Verification items for this drawing (mm, ordinates from the low corner). Coordinates: 2 decimals unless noted, no trailing zeros. Order: outer loops, then holes, each group sorted by start corner. A loop starts at its lowest first (then second) coordinate and runs counter-clockwise, first axis right, second up. Notation, with made-up numbers: M 40,-5 L 45,-5 A32 cw 45,23 Z; hole C -39.5,33 d7. An arc over 180 degrees is marked long. One line per item, written item: value. Start each with the question number.
1) Thickness scan on L1, parallel to Y at x = 50, z = 24.25; L2, parallel to Z at x = 108, y = 27.5; L3, parallel to Y at x = 17, z = 25. Record the ranges inside material, lowest first. Write a range as from..to.
2) Sectioned sample at B-B, the plane x = 170. Enter the section's corners in (y, z), then the cut area to 3 significant figures.
3) Sectioned sample at A-A, the plane y = 31. Enter the section's corners in (x, z), then the cut area to 3 significant figures.
4) Sectioned sample at C-C, the plane z = 25.75. Enter the section's corners in (x, y).
5) Sectioned sample at D-D, the plane x = 79. Enter the section's corners in (y, z), then the cut area to 3 significant figures.
6) Go/stop test with flat-tipped pins: P1, Ø23, axis at x = 50, y = 25, coming from the -Z side; P2, Ø6, axis at x = 168.5, y = 30, coming from the +Z side. Record where each tip stops, or that it passes through.
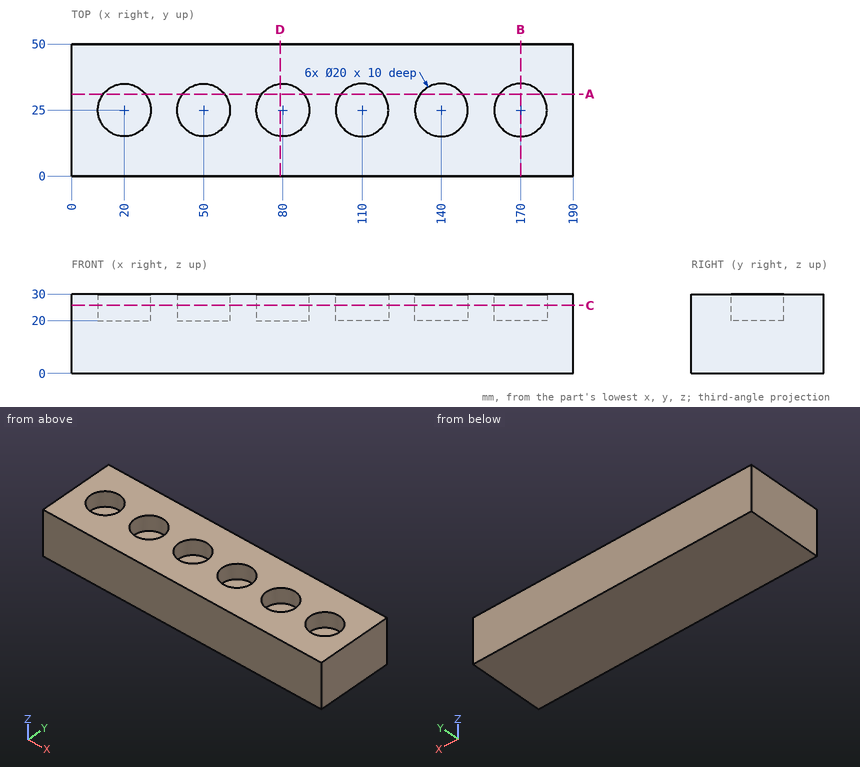
Final values:
1. L1: y = 0..15, 35..50
1. L2: z = 0..20
1. L3: y = 0..15.46, 34.54..50
2. outline: M 0,0 L 50,0 L 50,30 L 35,30 L 35,20 L 15,20 L 15,30 L 0,30 Z
2. area: 1,300 mm^2
3. outline: M 0,0 L 190,0 L 190,30 L 178,30 L 178,20 L 162,20 L 162,30 L 148,30 L 148,20 L 132,20 L 132,30 L 118,30 L 118,20 L 102,20 L 102,30 L 88,30 L 88,20 L 72,20 L 72,30 L 58,30 L 58,20 L 42,20 L 42,30 L 28,30 L 28,20 L 12,20 L 12,30 L 0,30 Z
3. area: 4,740 mm^2
4. outline: M 0,0 L 190,0 L 190,50 L 0,50 Z; hole C 20,25 d20; hole C 50,25 d20; hole C 80,25 d20; hole C 110,25 d20; hole C 140,25 d20; hole C 170,25 d20
5. outline: M 0,0 L 50,0 L 50,30 L 34.95,30 L 34.95,20 L 15.05,20 L 15.05,30 L 0,30 Z
5. area: 1,300 mm^2
6. P1: stops at z = 0
6. P2: stops at z = 20
